Could you check a few things on this model? Use its own coordinates, in mm. Coordinates: 2 decimals unless noted, no trailing zeros. Order: outer loops, then holes, each group sorted by start corner. A loop starts at its lowest first (then second) coordinate and runs counter-clockwise, first axis right, second up. Notation, with made-up numbers: M 37.25,-29.75 L 56.25,-29.75 A24 cw 56.25,8.25 Z; hole C 87.5,55 d5. An arc over 180 degrees is marked long. One line per question, with ' | ' between items. Start each with the question number.
from build123d import *

# Parameters (mm, degrees)
SKETCH1_W           = 192.07988
SKETCH1_H           = 66.04
SKETCH1_R           = 7
SKETCH1_R_2         = 12.7
SKETCH1_R_3         = 2.25
BOSS_EXTRUDE1_DEPTH = 3.175


with BuildPart() as part:
    # Sketch1 → Boss-Extrude1 (new body)
    with BuildSketch(Plane.YZ):
        Rectangle(SKETCH1_W, SKETCH1_H)
        with Locations(Location((63.01994, 0, 0), (0, 0, 270))):
            Circle(SKETCH1_R, mode=Mode.SUBTRACT)
        with Locations(Location((0, 0, 0), (0, 0, 270))):
            Circle(SKETCH1_R_2, mode=Mode.SUBTRACT)
        with Locations(Location((-79.831946, 28.02001, 0), (0, 0, 270))):
            Circle(SKETCH1_R_3, mode=Mode.SUBTRACT)
        with Locations(Location((-79.831946, -28.02001, 0), (0, 0, 270))):
            Circle(SKETCH1_R_3, mode=Mode.SUBTRACT)
        with Locations(Location((-46.207934, -28.02001, 0), (0, 0, 270))):
            Circle(SKETCH1_R_3, mode=Mode.SUBTRACT)
        with Locations(Location((-46.207934, 28.02001, 0), (0, 0, 270))):
            Circle(SKETCH1_R_3, mode=Mode.SUBTRACT)
    extrude(amount=BOSS_EXTRUDE1_DEPTH)


solid = part.part
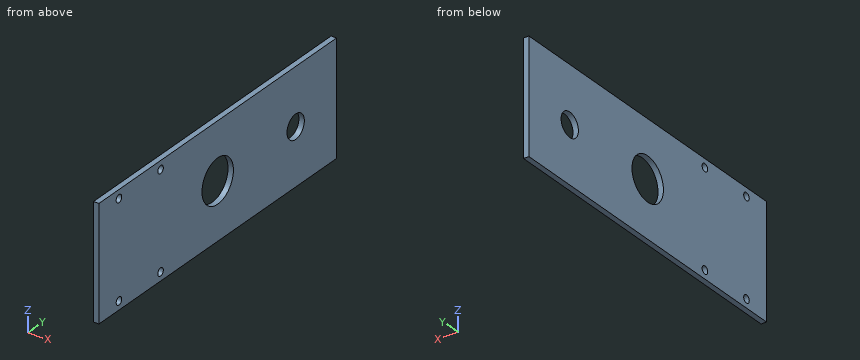
(1) Imagine slicing it at A-A, the plane z = 0. Write out the boundary of the cut face in (x, y) (3 decimals), plus the area to 3 significant figures.
(2) If I drill on line 1 along Y through (x, z) = (1.5, 0); line 2 along Y through (x, z) = (2, -26.5); line 3 along Z through (x, y) = (0.5, -79), over which ranges is the centre line in solid material (lowest first)? Write a range as from..to.
(3) Imagine slicing it at C-C, the plane x = 0.65. Write out the boundary of the cut face in (y, z), plus the area to 3 significant figures.
(4) Imagine slicing it at B-B, the plane y = 0. Write out the boundary of the cut face in (x, z) (3 decimals).
Answers:
1) outline: M 0,-96.04 L 3.175,-96.04 L 3.175,-12.7 L 0,-12.7 Z; M 0,12.7 L 3.175,12.7 L 3.175,56.02 L 0,56.02 Z; M 0,70.02 L 3.175,70.02 L 3.175,96.04 L 0,96.04 Z | area: 485 mm²
2) line 1: -96.04..-12.7, 12.7..56.02, 70.02..96.04 | line 2: -96.04..-81.49, -78.17..-47.87, -44.55..96.04 | line 3: -33.02..-30.11, -25.93..25.93, 30.11..33.02
3) outline: M -96.04,-33.02 L 96.04,-33.02 L 96.04,33.02 L -96.04,33.02 Z; hole C -79.83,-28.02 d4.5; hole C -79.83,28.02 d4.5; hole C -46.21,-28.02 d4.5; hole C -46.21,28.02 d4.5; hole C 0,0 d25.4; hole C 63.02,0 d14 | area: 12,000 mm²
4) outline: M 0,-33.02 L 3.175,-33.02 L 3.175,-12.7 L 0,-12.7 Z; M 0,12.7 L 3.175,12.7 L 3.175,33.02 L 0,33.02 Z
